Read the model definition and answer for the solid it produces. Units are mm, in the model's axes. Face numbers are marked on the shaded views. Coordinates: 2 decimals unless noted, no trailing zeros. Write each loop counter-clockwise with the first axis right and the second up, starting at its lowest first coordinate (ties: lowest second). Pieces come first, ordered by that corner, then holes. Notation, with made-up numbers: (50.25, -10) -> (94.25, -10) arc R35 cw to (94.25, 28) -> close; hole circle Ø5 at (88.5, 13). An arc over 180 degrees is marked (long way). Write item = value, one per line. Start each with the question number.
1) Section A-A (x = 0) is taken. Determine the outline of the cut face in (y, z) (3 decimals), plus the area to 3 significant figures.
2) Section D-D (x = 19.5) is taken. Determine the outline of the cut face in (y, z) (3 decimals), plus the area to 3 significant figures.
3) Section C-C (z = 10) is taken. Determine the outline of the cut face in (x, y) (3 decimals), plus the area to 3 significant figures.
4) Find the intervals of material crossed by line 1 along Z through (x, y) = (15, 7) (3 decimals); line 2 along X through (y, z) = (-1.5, 10), in increasing order. Write a range as from..to.
5) Flat-ended cylindrical pins translate along their axes: pin 1 Ø5 at (x, y) = (-1.5, -17) entering from +Z (3 decimals); pin 2 Ø6 at (x, y) = (27, 20.5) entering from -Z; pin 3 Ø3 at (y, z) = (-2.5, 11) entering from -X. Find the tip coordinate at first contact, or state that the pin passes through.
6) For a pull along Z with two mould halves and no side action, classify the marked faces 1, 2 and 3 as released by +Z, released by -Z, zero draft, split by the parting line, or undercut.
from build123d import *

# Parameters (mm, degrees)
F0_R     = 3.175
F1_DEPTH = 12.7
F2_W     = 76.2
F2_H     = 76.2
F3_DEPTH = 3.175


with BuildPart() as f1:
    # F0 (on Top) → F1 (new body)
    with BuildSketch(Plane.XY):
        Circle(F0_R)
    extrude(amount=F1_DEPTH)

    # F2 (on Top) → F3 (join)
    with BuildSketch(Plane.XY):
        Rectangle(F2_W, F2_H)
    extrude(amount=F3_DEPTH)


solid = f1.part
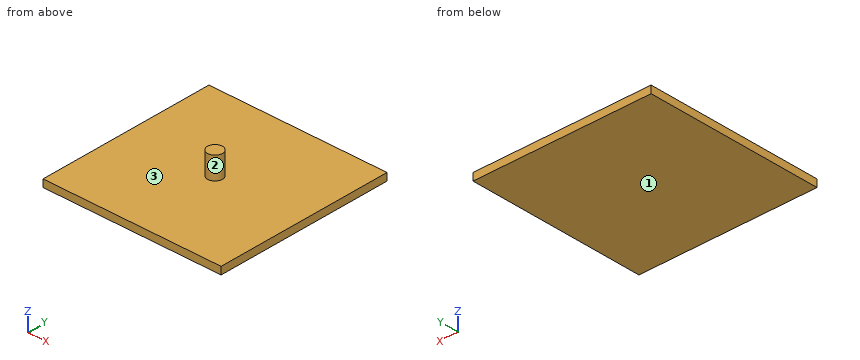
Answer key:
q1.outline = (-38.1, 0) -> (38.1, 0) -> (38.1, 3.175) -> (3.175, 3.175) -> (3.175, 12.7) -> (-3.175, 12.7) -> (-3.175, 3.175) -> (-38.1, 3.175) -> close
q1.area = 302 mm^2
q2.outline = (-38.1, 0) -> (38.1, 0) -> (38.1, 3.175) -> (-38.1, 3.175) -> close
q2.area = 242 mm^2
q3.outline = circle Ø6.35 at (0, 0)
q3.area = 31.7 mm^2
q4.line_1 = 0..3.175
q4.line_2 = -2.8..2.8
q5.pin_1 = 3.175
q5.pin_2 = 0
q5.pin_3 = -3.01
q6.face_1 = released by -Z
q6.face_2 = zero draft
q6.face_3 = released by +Z
